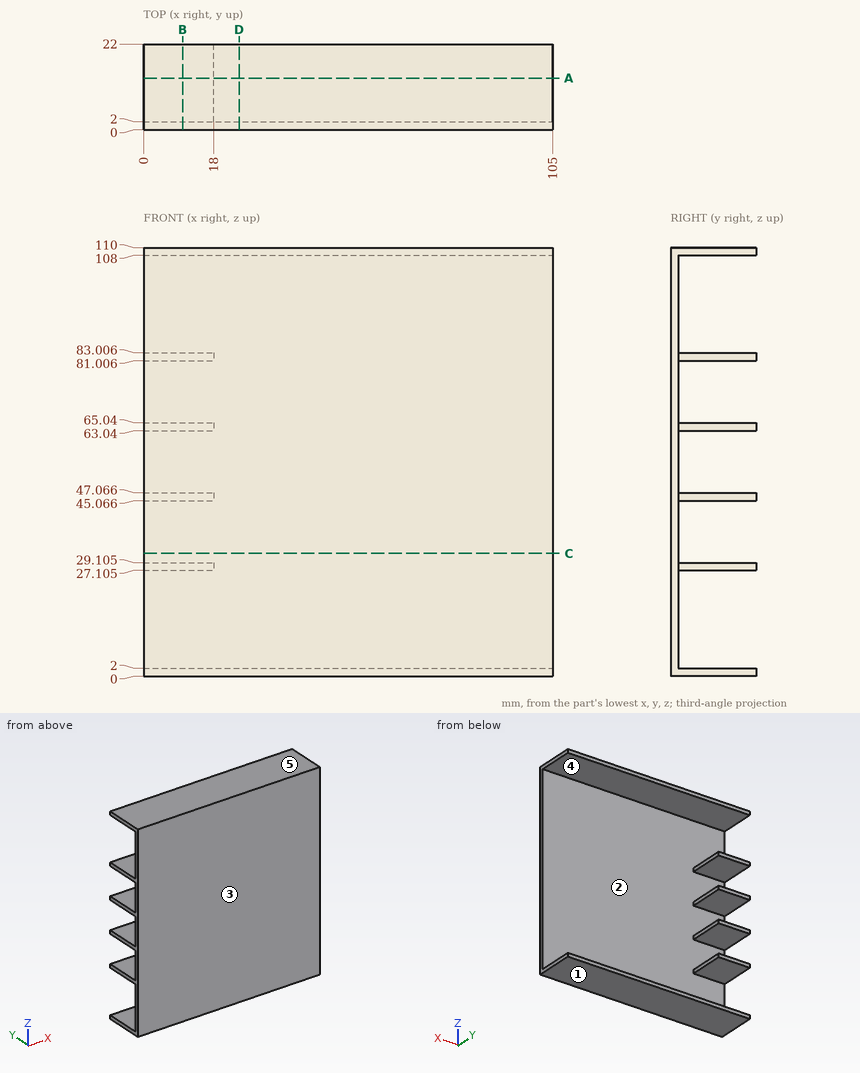
Print and shaded views of the part. All mm, measured from the part's lowest x, y and z. A direction names the side the tool comes from. Round coordinates to 2 decimals unless told otherwise and drop trailing zeros. Write each loop counter-clockwise with the first axis right and the second up, starting at its lowest first coordinate (ties: lowest second). Pieces come first, ordered by that corner, then holes. Notation, with made-up numbers: (65.5, -4) - (96.5, -4) arc R22 cw to (96.5, 18) - close; hole circle Ø8 at (39, -23.75). An arc over 180 degrees is marked (long way). One line per item, written item: value.
(1) Two-plate mould, pull along Z, no slides. Class the marked faces 1, 2 and 3: pulls with the +Z half, pulls with the -Z half, needs draft (parallel to the pull), parting line crosses it, or undercut.
Values follow:
face 1: pulls with the -Z half
face 2: undercut
face 3: needs draft
(2) 3-axis set-ups, long thin cutter, end or side, ignore diameter. For the marked faces 4 and 5: which of +Z, -Z, +X, -X, +Y, -Y reach the whole face in a straight line?
Values follow:
face 4: +X, -X, +Y
face 5: +Z, +X, -X, +Y, -Y
(3) Cut at A-A, the plane y = 13.25. Give the cut face in (x, z) (1 decimal), plus the area to 3 significant figures.
Values follow:
outline: (0, 0) - (105, 0) - (105, 2) - (0, 2) - close; (0, 27.1) - (18, 27.1) - (18, 29.1) - (0, 29.1) - close; (0, 45.1) - (18, 45.1) - (18, 47.1) - (0, 47.1) - close; (0, 63) - (18, 63) - (18, 65) - (0, 65) - close; (0, 81) - (18, 81) - (18, 83) - (0, 83) - close; (0, 108) - (105, 108) - (105, 110) - (0, 110) - close
area: 564 mm²
(4) Cut at D-D, the plane x = 24.5. Give the cut face in (y, z).
Values follow:
outline: (0, 0) - (22, 0) - (22, 2) - (2, 2) - (2, 108) - (22, 108) - (22, 110) - (0, 110) - close
(5) Drop flat-ended pins along their axis: P1, Ø2, axis at y = 12.5, z = 82.5, coming from the +X side; P2, Ø3, axis at x = 66.5, z = 16.5, coming from the +Y side. Give the stop position or say it passes through.
Values follow:
P1: stops at x = 18
P2: stops at y = 2
(6) Cut at C-C, the plane z = 31.5. Give the cut face in (x, y).
Values follow:
outline: (0, 0) - (105, 0) - (105, 2) - (0, 2) - close
(7) Wall check: probe 1 along Z at (x, y) = (9.5, 21) (1 decimal); probe 2 along Z at (x, y) = (70.5, 18.5); probe 3 along X at (y, z) = (4, 28). Give the ranges that are in metal, low to high.
Values follow:
probe 1: z = 0 to 2, 27.1 to 29.1, 45.1 to 47.1, 63 to 65, 81 to 83, 108 to 110
probe 2: z = 0 to 2, 108 to 110
probe 3: x = 0 to 18
(8) Cut at B-B, the plane x = 10. Give the cut face in (y, z) (1 decimal), plus the area to 3 significant figures.
Values follow:
outline: (0, 0) - (22, 0) - (22, 2) - (2, 2) - (2, 27.1) - (22, 27.1) - (22, 29.1) - (2, 29.1) - (2, 45.1) - (22, 45.1) - (22, 47.1) - (2, 47.1) - (2, 63) - (22, 63) - (22, 65) - (2, 65) - (2, 81) - (22, 81) - (22, 83) - (2, 83) - (2, 108) - (22, 108) - (22, 110) - (0, 110) - close
area: 460 mm²
